Part print with two shaded views. Sizes in mm from the minimum x, y, z corner. A direction names the side the tool comes from. Round coordinates to 2 decimals unless told otherwise and drop trailing zeros. Write each loop counter-clockwise with the first axis right and the second up, starting at its lowest first coordinate (ties: lowest second). Pieces come first, ordered by that corner, then holes. Notation, with made-up numbers: (-19, -29) - (29, -29) arc R32 cw to (29, 2) - close; hole circle Ø4 at (-39.75, 84). An arc over 180 degrees is marked (long way). Answer as a JSON object with one key per item and string values. Group by question number.
Item 1: Which spindle directions (+Z, -Z, +X, -X, +Y, -Y) get a long thin tool onto all of the face, cutting with end or side? Do the marked faces 1 and 2. Say none if no direction does.
Item 2: Slice it at A-A, the plane z = 9. List the corners of the cut face in (x, y) (3 decimals).
Item 3: Two-plate mould, pull along Z, no slides. Class the marked faces 3, 4 and 5: +Z half, -Z half, draft (parallel to the pull), parting line (faces both ways), or undercut.
Item 4: Flat gauge pins, fed straight in: pin 1 (1 mm diameter, centred on x = 27.5, y = 6.5, fed in from -Z); pin 2 (9 mm diameter, centred on x = 23, y = 27.5, fed in from -Z); pin 3 (19 mm diameter, centred on x = 28, z = 33, fed in from +Y); pin 4 (12 mm diameter, centred on x = 19, z = 33, fed in from +Y). Where does each tip first touch, or does it go through?
Item 5: Slice it at D-D, the plane y = 25. List the corners of the cut face in (x, z).
Item 6: Slice it at C-C, the plane x = 13. List the corners of the cut face in (y, z).
Item 7: Slice it at B-B, the plane y = 4. List the corners of the cut face in (x, z) (3 decimals).
Item 8: Probe line 1 (X direction, y = 5, z = 9) (3 decimals); line 2 (Y direction, x = 19, z = 45); line 3 (Z direction, x = 13, y = 31). List the from-to ranges inside material, lowest first. Write a range as from..to.
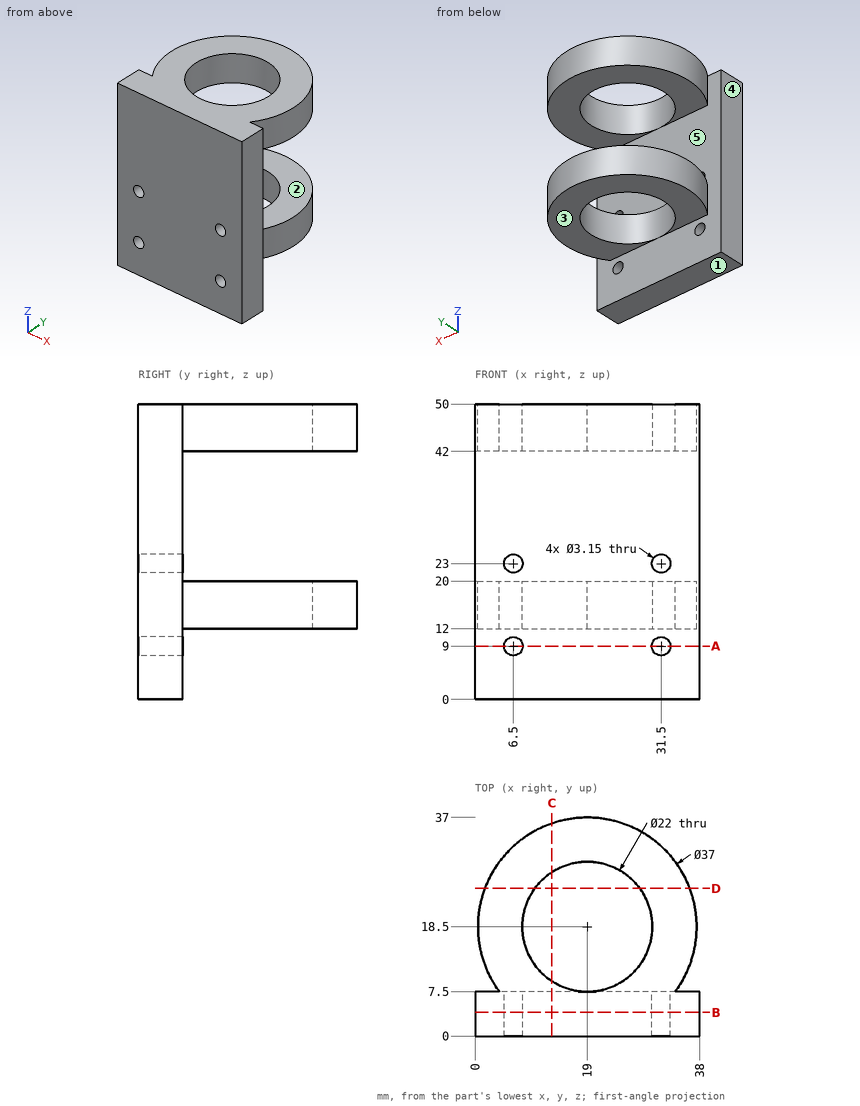
Geometry says:
{
 "1": {"face 1": "-Z, +X, -X, +Y, -Y", "face 2": "+X, -X, +Y"},
 "2": {"outline": "(0, 0) - (4.925, 0) - (4.925, 7.5) - (0, 7.5) - close; (8.075, 0) - (29.925, 0) - (29.925, 7.5) - (8.075, 7.5) - close; (33.075, 0) - (38, 0) - (38, 7.5) - (33.075, 7.5) - close"},
 "3": {"face 3": "-Z half", "face 4": "draft", "face 5": "undercut"},
 "4": {"pin 1": "stops at z = 0", "pin 2": "stops at z = 12", "pin 3": "stops at y = 36.01", "pin 4": "stops at y = 7.5"},
 "5": {"outline": "(1.68, 12) - (10.13, 12) - (10.13, 20) - (1.68, 20) - close; (1.68, 42) - (10.13, 42) - (10.13, 50) - (1.68, 50) - close; (27.87, 12) - (36.32, 12) - (36.32, 20) - (27.87, 20) - close; (27.87, 42) - (36.32, 42) - (36.32, 50) - (27.87, 50) - close"},
 "6": {"outline": "(0, 0) - (7.5, 0) - (7.5, 12) - (9.28, 12) - (9.28, 20) - (7.5, 20) - (7.5, 42) - (9.28, 42) - (9.28, 50) - (0, 50) - close; (27.72, 12) - (36, 12) - (36, 20) - (27.72, 20) - close; (27.72, 42) - (36, 42) - (36, 50) - (27.72, 50) - close"},
 "7": {"outline": "(0, 0) - (38, 0) - (38, 50) - (0, 50) - close; hole circle Ø3.15 at (6.5, 9); hole circle Ø3.15 at (6.5, 23); hole circle Ø3.15 at (31.5, 9); hole circle Ø3.15 at (31.5, 23)"},
 "8": {"line 1": "x = 0..4.925, 8.075..29.925, 33.075..38", "line 2": "y = 0..7.5, 29.5..37", "line 3": "z = 12..20, 42..50"}
}
